Work out the finished part from the listing and answer in its coordinate system (mm). A direction names the side the tool comes from. Coordinates: 2 decimals unless noted, no trailing zeros. Order: outer loops, then holes, each group sorted by start corner. A loop starts at its lowest first (then second) coordinate and runs counter-clockwise, first axis right, second up. Notation, with made-up numbers: (46, 87) - (51, 87) arc R22 ccw to (51, 119) - close; hole circle Ø2 at (61.5, 35.25). An arc over 180 degrees is marked (long way). Use CSV: the item, a comma, the result in double quotes. Start each with the question number.
from build123d import *

# Parameters (mm, degrees)
EXTRUDE_1_DEPTH      = 6
SKETCH_2_W           = 7
SKETCH_2_H           = 6
EXTRUDE_2_DEPTH      = 6
CUT_EXTRUDE_1_DEPTH  = 7
SKETCH_21_W          = 7
SKETCH_21_H          = 6
EXTRUDE_21_DEPTH     = 6
CUT_EXTRUDE_11_DEPTH = 7


with BuildPart() as part:
    # Эскиз1 → Бобышка-Вытянуть1 (new body)
    with BuildSketch(Plane.XY):
        with BuildLine():
            Line((81, -293.846153846), (81, -307.846153846))
            ThreePointArc((81, -307.846153846), (80.327690782, -310.350368792), (78.491563001, -312.181141022))
            Line((78.491563001, -312.181141022), (6, -353.846153846))
            Line((6, -353.846153846), (6, -293.846153846))
            Line((6, -293.846153846), (81, -293.846153846))
        make_face()
    extrude(amount=-EXTRUDE_1_DEPTH)

    # Эскиз2 → Бобышка-Вытянуть2 (add)
    with BuildSketch(Plane(origin=(56, -310.846153846, 0), x_dir=(0, 1, 0), z_dir=(0, 0, 1))):
        with Locations((-9.531849908, 53)):
            Rectangle(SKETCH_2_W, SKETCH_2_H)
        with Locations((9.531849908, 53)):
            Rectangle(SKETCH_2_W, SKETCH_2_H)
    extrude(amount=-EXTRUDE_2_DEPTH)

    # Эскиз3 → Вырез-Вытянуть1 (cut, through all)
    with BuildSketch(Plane(origin=(56, -310.846153846, 0), x_dir=(0, 1, 0), z_dir=(0, 0, 1))):
        Polygon((-2.1, 42), (-3.6, 42), (-3.6, 39.6), (-2.1, 39.6), (-2.1, 35), (2.1, 35), (2.1, 39.6), (3.6, 39.6), (3.6, 42), (2.1, 42), (2.1, 50), (-2.1, 50), align=None)
    extrude(amount=-CUT_EXTRUDE_1_DEPTH, mode=Mode.SUBTRACT)

    # Эскиз21 → Бобышка-Вытянуть21 (add)
    with BuildSketch(Plane(origin=(48, -343.846153846, 0), x_dir=(1, 0, 0), z_dir=(0, 0, 1))):
        with Locations((-9.531849908, 53)):
            Rectangle(SKETCH_21_W, SKETCH_21_H)
        with Locations((9.531849908, 53)):
            Rectangle(SKETCH_21_W, SKETCH_21_H)
    extrude(amount=-EXTRUDE_21_DEPTH)

    # Эскиз31 → Вырез-Вытянуть11 (cut, through all)
    with BuildSketch(Plane(origin=(48, -343.846153846, 0), x_dir=(1, 0, 0), z_dir=(0, 0, 1))):
        Polygon((-2.1, 42), (-3.6, 42), (-3.6, 39.6), (-2.1, 39.6), (-2.1, 35), (2.1, 35), (2.1, 39.6), (3.6, 39.6), (3.6, 42), (2.1, 42), (2.1, 50), (-2.1, 50), align=None)
    extrude(amount=-CUT_EXTRUDE_11_DEPTH, mode=Mode.SUBTRACT)


solid = part.part
1) The part is cut by section D-D on x = 27. Determine the outline of the cut face in (y, z), plus the area to 3 significant figures.
2) Straight lines are drawn through the part: line 1 (X direction, y = -295.5, z = -3.2); line 2 (X direction, y = -302.5, z = -3); line 3 (X direction, y = -308.5, z = -2.4). For each, find the intervals that lie inside material, in ascending order. Write a range as [from, to].
3) The part is cut by section C-C on y = -326. Determine the outline of the cut face in (x, z).
4) For a pull along Y with two mould halves and no side action, classify faces 1 (the face through (15, -307.246, -3)), 2 (the face through (6, -307, -3)), 3 (the face through (41, -313, 0)), 4 (the face through (44, -293.846, -3)) as +Y half, -Y half, draft (parallel to the pull), parting line (faces both ways), or undercut.
5) The part is cut by section A-A on y = -293. Determine the outline of the cut face in (x, z).
6) Flat-ended cylindrical pins translate along their axes: P1, Ø1, axis at y = -326, z = -2, coming from the -X side; P2, Ø3, axis at y = -297, z = -5, coming from the -X side; P3, Ø0.7, axis at x = 15, z = -2.5, coming from the -Y side; P4, Ø1.2, axis at y = -313.5, z = -2.5, coming from the +X side. Find the tip coordinate at first contact, or state that the pin passes through.
7) For faces 5 (the face through (48, -308.846, -3)), 6 (the face through (10, -308.746, -3)), 7 (the face through (61.032, -291, -3)), 8 (the face through (20, -293.846, -3)), determine the directions among +Z, -Z, +X, -X, +Y, -Y from which every point of the face is accessible in a straight line to the end or side of a thin tool.
8) The part is cut by section B-B on x = 13. Determine the outline of the cut face in (y, z).
Answer key:
1,outline,"(-341.78, -6) - (-293.85, -6) - (-293.85, 0) - (-341.78, 0) - close"
1,area,"288 mm^2"
2,line 1,"[6, 45.9], [50.1, 81]"
2,line 2,"[0, 44.4], [51.6, 81]"
2,line 3,"[6, 14], [16.4, 45.9], [50.1, 80.96]"
3,outline,"(6, -6) - (54.45, -6) - (54.45, 0) - (6, 0) - close"
4,face 1,"undercut"
4,face 2,"undercut"
4,face 3,"draft"
4,face 4,"+Y half"
5,outline,"(34.97, -6) - (41.97, -6) - (41.97, 0) - (34.97, 0) - close; (54.03, -6) - (61.03, -6) - (61.03, 0) - (54.03, 0) - close"
6,P1,"x = 6"
6,P2,"x = 0"
6,P3,"y = -348.87"
6,P4,"x = 77.24"
7,face 5,"+Z, -Z, +Y"
7,face 6,"+Z, -Z, -X"
7,face 7,"+Z, -Z, +X, +Y"
7,face 8,"+Z, -Z, -X, +Y"
8,outline,"(-349.82, -6) - (-312.95, -6) - (-312.95, 0) - (-349.82, 0) - close; (-308.75, -6) - (-293.85, -6) - (-293.85, 0) - (-308.75, 0) - close"
